from build123d import *

# Parameters (mm, degrees)
PAD003_DEPTH    = 1.42
POCKET004_DEPTH = 8.875
POCKET005_DEPTH = 8.570714
CHAMFER002_SIZE = 0.5


with BuildPart() as part:
    # Sketch010 → Pad003 (new body)
    with BuildSketch(Plane.XZ):
        Polygon((-4.284857, 0), (4.284857, 0), (4.284857, 8.875), (4.284857, 35.5), (-4.284857, 35.5), (-4.284857, 8.875), align=None)
    extrude(amount=PAD003_DEPTH)

    # Sketch011 (on Face1 of Pad003) → Pocket004 (cut)
    with BuildSketch(Plane(origin=(0, 0, 0), x_dir=(1, 0, 0), z_dir=(0, 0, -1))):
        Polygon((-3.284857, 1.42), (-3.284857, 1), (-8.284857, 1), (-8.284857, 4.921038), align=None)
        Polygon((8.284857, 4.921038), (3.284857, 1.42), (3.284857, 1), (8.284857, 1), align=None)
    extrude(amount=-POCKET004_DEPTH, mode=Mode.SUBTRACT)

    # Sketch012 (on Face9 of Pocket004) → Pocket005 (cut, through all)
    with BuildSketch(Plane(origin=(-4.284857, 0, 0), x_dir=(0, 0, -1), z_dir=(-1, 0, 0))):
        Polygon((-39.051991, 0.19), (-10.038814, 1.44), (-39.051991, 14.02), align=None)
    extrude(amount=-POCKET005_DEPTH, mode=Mode.SUBTRACT)

    # Chamfer002
    chamfer002_edges = [part.edges().sort_by_distance(p)[0] for p in [
        (-3.784857, -1, 0),
        (-3.284857, -1.21, 0),
        (0, -1.42, 0),
        (3.284857, -1.21, 0),
        (3.784857, -1, 0),
        (-4.284857, -0.5, 0),
        (4.284857, -0.5, 0),
    ]]
    chamfer(chamfer002_edges, length=CHAMFER002_SIZE)


with BuildPart() as part_1:
    # Body001 placement: moved
    add(part.part.moved(Location((0, 25, 0))))


solid = part_1.part
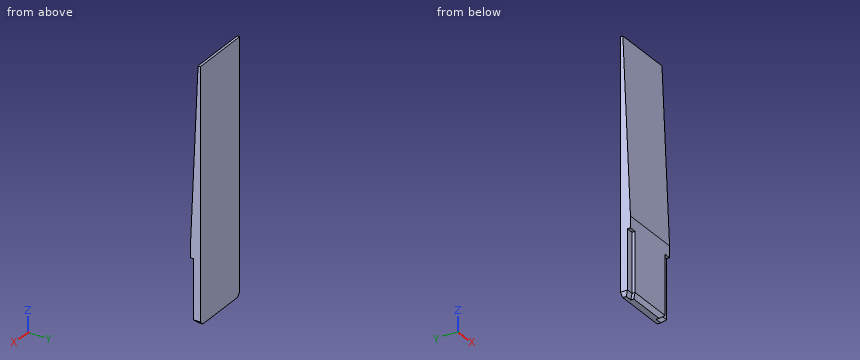
The model under review builds one solid part; all positions refer to its coordinate system, in mm. Round coordinates to 2 decimals unless told otherwise and drop trailing zeros. Order: outer loops, then holes, each group sorted by start corner. A loop starts at its lowest first (then second) coordinate and runs counter-clockwise, first axis right, second up. Notation, with made-up numbers: (-0.5, 86.5) - (43.5, 86.5) arc R17 cw to (43.5, 114.5) - close; hole circle Ø2 at (0, -17). An arc over 180 degrees is marked (long way). Use one line per item in the form item = value.
Q1. Add section B-B on x = 1. Give the boundary of the cut face in (y, z).
Response values:
outline = (23.58, 0.5) - (24.08, 0) - (25, 0) - (25, 35.5) - (24.66, 35.5) - (23.58, 10.5) - close
Q2. To check wall thickness, follow line 1 (X direction, y = 23.7, z = 5); line 2 (Y direction, x = 3.5, z = 1.5); line 3 (Y direction, x = -2.75, z = 28). State the ranges of each line that lie inside material, in increasing order.
Response values:
line_1 = -3.28 to 3.28
line_2 = 24 to 25
line_3 = 24.33 to 25
Q3. Clearance check with flat-ended pins moving along their axes: P1, Ø1.1, axis at x = 3.5, z = 3.5, coming from the -Y side; P2, Ø0.5, axis at x = -3.5, y = 24, coming from the -Z side. State where each tip first meets the part, or that it passes through.
Response values:
P1 = 23.58
P2 = 0.25
Q4. Add section D-D on z = 25.5. Give the boundary of the cut face in (x, y), then the cut area to 3 significant figures.
Response values:
outline = (-4.28, 24.23) - (4.28, 24.23) - (4.28, 25) - (-4.28, 25) - close
area = 6.63 mm^2
Q5. Add section A-A on z = 7.5. Give the boundary of the cut face in (x, y), then the cut area to 3 significant figures.
Response values:
outline = (-4.28, 24) - (-3.28, 24) - (-3.28, 23.58) - (3.28, 23.58) - (3.28, 24) - (4.28, 24) - (4.28, 25) - (-4.28, 25) - close
area = 11.3 mm^2
Q6. Add section C-C on z = 15. Give the boundary of the cut face in (x, y), then the cut area to 3 significant figures.
Response values:
outline = (-4.28, 23.77) - (4.28, 23.77) - (4.28, 25) - (-4.28, 25) - close
area = 10.5 mm^2
